Design review of the part built by this model. Coordinates are the model's own, in mm. Face numbers are marked on the shaded views. A direction names the side the tool comes from. Coordinates: 2 decimals unless noted, no trailing zeros. Write each loop counter-clockwise with the first axis right and the second up, starting at its lowest first coordinate (ties: lowest second). Pieces come first, ordered by that corner, then holes. Notation, with made-up numbers: (-31.5, 84) -> (-2.5, 84) arc R23 cw to (-2.5, 103) -> close; hole circle Ø8 at (-13.5, -8). An arc over 180 degrees is marked (long way). Answer in a Markdown table with one row per item. Add a question column.
Item 1: Take a section at C-C, the plane y = 46.5. Write out the cut boundary in (x, z).
Item 2: Clearance check with flat-ended pins moving along their axes: P1, Ø5, axis at x = 14, y = 26.5, coming from the +Z side; P2, Ø1.2, axis at y = 15.5, z = 10.25, coming from the -X side; P3, Ø6, axis at x = 18, z = 10.5, coming from the -Y side; P4, Ø2, axis at x = 4, z = 5.5, coming from the +Y side. State where each tip first meets the part, or that it passes through.
Item 3: Take a section at A-A, the plane y = 57. Write out the cut boundary in (x, z) (3 decimals).
Item 4: For the marked faces 1, 2 and 3, list the 3-axis set-ups (+Z, -Z, +X, -X, +Y, -Y) from which the entire face can be reached by the end or side of a thin tool; tool diameter is ignored.
Item 5: To check wall thickness, follow line 1 (X direction, y = 6, z = 1.5); line 2 (Y direction, x = 29.5, z = 13.75); line 3 (X direction, y = 32.5, z = 8.75). State the ranges of each line that lie inside material, in increasing order.
Item 6: Take a section at D-D, the plane y = 11. Write out the cut boundary in (x, z), and give its area (3 significant figures).
Item 7: Take a section at B-B, the plane z = 5.25. Write out the cut boundary in (x, y), and give its area (3 significant figures).
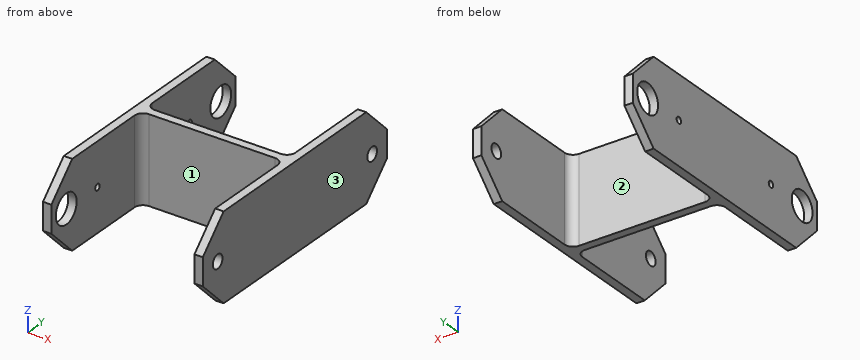
from build123d import *

# Parameters (mm, degrees)
F1_DEPTH = 20.5
F2_SIZE  = 7
F3_R     = 3.5
F3_R_2   = 0.75
F4_DEPTH = 25
F5_R     = 1.625
F6_DEPTH = 25
F9_R     = 2


with BuildPart() as f1:
    # F0 (on Top) → F1 (new body)
    with BuildSketch(Plane.XY):
        Polygon((-2, 0), (0, 0), (0, 30), (34, 30), (34, 0), (36, 0), (36, 32), (-2, 32), align=None)
    extrude(amount=F1_DEPTH)

    # F2
    f2_edges = [f1.edges().sort_by_distance(p)[0] for p in [
        (-1, 0, 0),
        (-1, 0, 20.5),
        (35, 0, 0),
        (35, 0, 20.5),
    ]]
    chamfer(f2_edges, length=F2_SIZE)

    # F3 (on face) → F4 (cut)
    with BuildSketch(Plane(origin=(-2, 0, 0), x_dir=(0, -1, 0), z_dir=(-1, 0, 0))):
        with Locations((-5, 10.25)):
            Circle(F3_R)
        with Locations((-15.5, 10.25)):
            Circle(F3_R_2)
    extrude(amount=-F4_DEPTH, mode=Mode.SUBTRACT)

    # F5 (on face) → F6 (cut)
    with BuildSketch(Plane.YZ.offset(36)):
        with Locations((5, 10.25)):
            Circle(F5_R)
    extrude(amount=-F6_DEPTH, mode=Mode.SUBTRACT)

    # F8: F1 across plane


with BuildPart() as f1_1:
    add(f1.part)
    add(f1.part.mirror(Plane(origin=(17, 31, 10.25), x_dir=(-1, 0, 0), z_dir=(0, 1, 0))))

    # F9
    f9_edges = [f1_1.edges().sort_by_distance(p)[0] for p in [
        (0, 30, 10.25),
        (0, 32, 10.25),
        (34, 32, 10.25),
        (34, 30, 10.25),
    ]]
    fillet(f9_edges, radius=F9_R)


solid = f1_1.part
Answers:
| question | item | result |
|---|---|---|
| 1 | outline | (-2, 0) -> (0, 0) -> (0, 9.5) -> (-2, 9.5) -> close; (-2, 11) -> (0, 11) -> (0, 20.5) -> (-2, 20.5) -> close; (34, 0) -> (36, 0) -> (36, 20.5) -> (34, 20.5) -> close |
| 2 | P1 | passes through |
| 2 | P2 | stops at x = 34 |
| 2 | P3 | stops at y = 30 |
| 2 | P4 | stops at y = 32 |
| 3 | outline | (-2, 2) -> (0, 2) -> (0, 6.75) -> (-2, 6.75) -> close; (-2, 13.75) -> (0, 13.75) -> (0, 18.5) -> (-2, 18.5) -> close; (34, 2) -> (36, 2) -> (36, 8.625) -> (34, 8.625) -> close; (34, 11.875) -> (36, 11.875) -> (36, 18.5) -> (34, 18.5) -> close |
| 4 | face 1 | +Z, -Z, -Y |
| 4 | face 2 | +Z, -Z, +Y |
| 4 | face 3 | +Z, -Z, +X, +Y, -Y |
| 5 | line 1 | x = -2 to 0, 34 to 36 |
| 5 | line 2 | y = 30 to 32 |
| 5 | line 3 | x = -2 to 0.68, 33.32 to 36 |
| 6 | outline | (-2, 0) -> (0, 0) -> (0, 20.5) -> (-2, 20.5) -> close; (34, 0) -> (36, 0) -> (36, 20.5) -> (34, 20.5) -> close |
| 6 | area | 82.0 mm^2 |
| 7 | outline | (-2, 1.75) -> (0, 1.75) -> (0, 28) arc R2 cw to (2, 30) -> (32, 30) arc R2 cw to (34, 28) -> (34, 1.75) -> (36, 1.75) -> (36, 60.25) -> (34, 60.25) -> (34, 34) arc R2 cw to (32, 32) -> (2, 32) arc R2 cw to (0, 34) -> (0, 60.25) -> (-2, 60.25) -> close |
| 7 | area | 305 mm^2 |
